Autodesk Inventor part; units mm, degrees
ref_plane "YZ Plane" through (0, 0, 0) normal (1, 0, 0) x (0, 1, 0)
ref_plane "XZ Plane" through (0, 0, 0) normal (0, 1, 0) x (-1, 0, 0)
ref_plane "XY Plane" through (0, 0, 0) normal (0, 0, 1) x (1, 0, 0)
sketch "Sketch1" plane through (0, 0, 0) normal (1, 0, 0) x (0, 1, 0)
  line L0 (0, 0) -> (321.6656, 0)
  line L1 (321.6656, 0) -> (321.6656, 321.6656)
  line L2 (321.6656, 321.6656) -> (0, 321.6656)
  line L3 (0, 321.6656) -> (0, 0)
  dimension "d0" = 321.6656
  dimension "d1" = 321.6656
extrude "Extrusion1" add sketch "Sketch1" along normal blind 4.7752
sketch "Sketch3" plane through (0, 0, 0) normal (-1, 0, 0) x (0, 0, 1)
  line L0 (0, 321.6656) -> (321.6656, 321.6656)
  line L1 (321.6656, 321.6656) -> (321.6656, 0)
  line L2 (0, 321.6656) -> (321.6656, 321.6656)
  line L3 (321.6656, 321.6656) -> (283.5656, 321.6656)
  line L4 (283.5656, 321.6656) -> (283.5656, 283.5656)
  line L5 (283.5656, 283.5656) -> (321.6656, 283.5656)
  line L6 (321.6656, 283.5656) -> (321.6656, 321.6656)
  line L7 (321.6656, 321.6656) -> (321.6656, 0)
  line L8 (321.6656, 0) -> (283.5656, 0)
  line L9 (283.5656, 0) -> (283.5656, 38.1)
  line L10 (283.5656, 38.1) -> (321.6656, 38.1)
  line L11 (321.6656, 38.1) -> (321.6656, 0)
  line L12 (321.6656, 0) -> (0, 0)
  line L13 (0, 0) -> (38.1, 0)
  line L14 (38.1, 0) -> (38.1, 38.1)
  line L15 (38.1, 38.1) -> (0, 38.1)
  line L16 (0, 38.1) -> (0, 0)
  line L17 (0, 321.6656) -> (38.1, 321.6656)
  line L18 (38.1, 321.6656) -> (38.1, 283.5656)
  line L19 (38.1, 283.5656) -> (0, 283.5656)
  line L20 (0, 283.5656) -> (0, 321.6656)
  line L21 (283.5656, 321.6656) -> (38.1, 321.6656)
  line L22 (38.1, 321.6656) -> (38.1, 283.5656)
  line L23 (38.1, 283.5656) -> (283.5656, 283.5656)
  line L24 (283.5656, 283.5656) -> (283.5656, 321.6656)
  line L25 (321.6656, 283.5656) -> (283.5656, 283.5656)
  line L26 (283.5656, 283.5656) -> (283.5656, 38.1)
  line L27 (283.5656, 38.1) -> (321.6656, 38.1)
  line L28 (321.6656, 38.1) -> (321.6656, 283.5656)
  line L29 (38.1, 38.1) -> (0, 38.1)
  line L30 (0, 38.1) -> (0, 283.5656)
  line L31 (0, 283.5656) -> (38.1, 283.5656)
  line L32 (38.1, 283.5656) -> (38.1, 38.1)
  line L33 (38.1, 38.1) -> (283.5656, 38.1)
  line L34 (283.5656, 38.1) -> (283.5656, 0)
  line L35 (283.5656, 0) -> (38.1, 0)
  line L36 (38.1, 0) -> (38.1, 38.1)
  line L37 (321.6656, 283.5656) -> (283.5656, 245.4656)
  line L38 (321.6656, 283.5656) -> (375.5471, 283.5656) construction
  line L39 (283.5656, 245.4656) -> (283.5656, 321.6656)
  line L40 (283.5656, 321.6656) -> (245.4656, 283.5656)
  line L41 (283.5656, 321.6656) -> (337.4471, 321.6656) construction
  line L42 (38.1, 321.6656) -> (76.2, 283.5656)
  line L43 (38.1, 321.6656) -> (91.9815, 321.6656) construction
  line L44 (0, 283.5656) -> (38.1, 245.4656)
  line L45 (0, 283.5656) -> (53.8815, 283.5656) construction
  line L46 (0, 38.1) -> (38.1, 76.2)
  line L47 (0, 38.1) -> (53.8815, 38.1) construction
  line L48 (38.1, 0) -> (76.2, 38.1)
  line L49 (38.1, 0) -> (91.9815, 0) construction
  line L50 (321.6656, 38.1) -> (283.5656, 76.2)
  line L51 (321.6656, 38.1) -> (375.5471, 38.1) construction
  line L52 (283.5656, 0) -> (245.4656, 38.1)
  line L53 (283.5656, 0) -> (337.4471, 0) construction
  dimension "d14" = 38.1
  dimension "d15" = 38.1
  dimension "d16" = 38.1
  dimension "d17" = 38.1
  dimension "d18" = 38.1
  dimension "d19" = 38.1
  dimension "d20" = 38.1
  dimension "d21" = 135
  dimension "d22" = 135
  dimension "d25" = 45
  dimension "d26" = 45
  dimension "d27" = 45
  dimension "d28" = 45
  dimension "d29" = 135
  dimension "d30" = 135
extrude "Extrusion4" cut sketch "Sketch3" against normal blind 4.7752 contours L0 L40 L23 L42 | L44 L32 L46 L30 | L1 L50 L26 L37 | L48 L33 L52 L12
sketch "Sketch4" plane through (0, 0, 0) normal (-1, 0, 0) x (0, 0, 1)
  line L0 (321.6656, 0) -> (283.5656, 0)
  line L1 (321.6656, 38.1) -> (321.6656, 0)
  line L2 (321.6656, 321.6656) -> (321.6656, 283.5656)
  line L3 (283.5656, 321.6656) -> (321.6656, 321.6656)
  line L4 (0, 321.6656) -> (38.1, 321.6656)
  line L5 (0, 283.5656) -> (0, 321.6656)
  line L6 (0, 0) -> (0, 38.1)
  line L7 (38.1, 0) -> (0, 0)
  line L8 (245.4656, 283.5656) -> (283.5656, 321.6656)
  line L9 (283.5656, 321.6656) -> (321.6656, 283.5656)
  line L10 (0, 283.5656) -> (0, 321.6656)
  line L11 (38.1, 321.6656) -> (0, 283.5656)
  line L12 (0, 38.1) -> (38.1, 0)
  line L13 (283.5656, 0) -> (321.6656, 38.1)
extrude "Extrusion5" cut sketch "Sketch4" against normal blind 4.7752
fillet "Fillet1" radius 6.35 16 edges at (2.3876, 283.5656, 0) (2.3876, 321.6656, 38.1) (2.3876, 38.1, 0) (2.3876, 76.2, 38.1) (2.3876, 0, 38.1) (2.3876, 283.5656, 76.2) (2.3876, 283.5656, 245.4656) (2.3876, 321.6656, 283.5656) (2.3876, 283.5656, 321.6656) (2.3876, 76.2, 283.5656) (2.3876, 245.4656, 283.5656) (2.3876, 0, 283.5656) (2.3876, 38.1, 321.6656) (2.3876, 38.1, 76.2) (2.3876, 38.1, 245.4656) (2.3876, 245.4656, 38.1)
sketch "Sketch6" plane through (0, 0, 0) normal (-1, 0, 0) x (0, 0, 1)
  circle A0 centre (-6.7619, -6.7309) radius 6.35
  circle A1 centre (71.9016, 17.9648) radius 6.35
  circle A2 centre (-24.7224, -24.6915) radius 6.35
  circle A3 centre (18.3502, 71.9326) radius 6.35
  circle A4 centre (39.0622, 11.5317) radius 2.159
  circle A5 centre (45.6554, 18.406) radius 2.159
  circle A6 centre (18.4365, 45.0628) radius 2.159
  circle A7 centre (32.185, 31.8764) radius 2.159
  circle A8 centre (11.8433, 38.1885) radius 2.159
  arc A9 (79.2947, 3.1748) -> (87.7766, 8.3381) centre (85.2874, 2.8788) ccw
  line L0 (87.7766, 28.6693) -> (87.7766, 8.3381)
  arc A10 (87.7766, 28.6693) -> (79.2947, 33.8326) centre (85.2874, 34.1286) ccw
  line L1 (40.1516, 33.8326) -> (79.2947, 33.8326)
  arc A11 (33.8016, 40.1826) -> (40.1516, 33.8326) centre (40.1516, 40.1826) ccw
  line L2 (33.8016, 79.3257) -> (33.8016, 40.1826)
  arc A12 (33.8016, 79.3257) -> (28.6383, 87.8076) centre (34.0976, 85.3184) ccw
  line L3 (28.6383, 87.8076) -> (8.3071, 87.8076)
  arc A13 (8.3071, 87.8076) -> (3.1438, 79.3257) centre (2.8478, 85.3184) ccw
  line L4 (3.1438, 27.4834) -> (3.1438, 79.3257)
  arc A14 (1.284, 22.9933) -> (3.1438, 27.4834) centre (-3.2062, 27.4834) ccw
  line L5 (-40.7893, -19.08) -> (1.284, 22.9933)
  arc A15 (-28.7596, -43.1049) -> (-19.111, -40.7583) centre (-23.1391, -45.2051) ccw
  line L6 (22.9623, 1.3149) -> (-19.111, -40.7583)
  arc A16 (27.4524, 3.1748) -> (22.9623, 1.3149) centre (27.4524, -3.1752) ccw
  line L7 (79.2947, 3.1748) -> (27.4524, 3.1748)
  circle A17 centre (85.2874, 34.1286) radius 2.95
  circle A18 centre (2.8478, 85.3184) radius 2.95
  circle A19 centre (-23.1391, -45.2051) radius 2.95
  circle A20 centre (85.2874, 2.8788) radius 2.95
  circle A21 centre (34.0976, 85.3184) radius 2.95
  point P0 (0, 0)
  point P1 (36.9766, 87.8076)
  dimension "d65" = 4.318
extrude "Extrusion7" cut sketch "Sketch6" against normal blind 25.4 contours A4 | A5 | A6 | A7 | A8
sketch "Sketch7" plane through (4.7752, 0, 0) normal (1, 0, 0) x (0, 0, -1)
  circle A0 centre (-31.8764, 289.4806) radius 2.159
  circle A1 centre (-11.5317, 282.6034) radius 2.159
  circle A2 centre (-38.1885, 309.8223) radius 2.159
  circle A3 centre (-18.406, 276.0102) radius 2.159
  circle A4 centre (-45.0628, 303.2291) radius 2.159
  circle A5 centre (-81.9118, 239.7538) radius 19.05
  line L0 (-38.1, 78.8303) -> (-38.1, 242.8353)
  arc A6 (-36.2401, 247.3255) -> (-38.1, 242.8353) centre (-31.75, 242.8353) ccw
  line L1 (-36.2401, 247.3255) -> (-4.4901, 279.0755)
  arc A7 (-4.4901, 279.0755) -> (-4.4901, 288.0557) centre (-8.9803, 283.5656) ccw
  line L2 (-4.4901, 288.0557) -> (-33.6099, 317.1755)
  arc A8 (-33.6099, 317.1755) -> (-42.5901, 317.1755) centre (-38.1, 312.6853) ccw
  line L3 (-42.5901, 317.1755) -> (-74.3401, 285.4255)
  arc A9 (-78.8303, 283.5656) -> (-74.3401, 285.4255) centre (-78.8303, 289.9156) ccw
  line L4 (-78.8303, 283.5656) -> (-242.8353, 283.5656)
  point P0 (0, 0)
  point P1 (-61.0348, 364.3954)
extrude "Extrusion8" cut sketch "Sketch7" against normal blind 25.4 contours A0 | A1 | A2 | A3 | A4
sketch "Sketch8" plane through (4.7752, 0, 0) normal (1, 0, 0) x (0, 0, -1)
  circle A0 centre (-289.7892, 32.185) radius 2.159
  circle A1 centre (-310.1339, 39.0622) radius 2.159
  circle A2 centre (-276.6028, 18.4365) radius 2.159
  circle A3 centre (-303.2596, 45.6554) radius 2.159
  circle A4 centre (-283.4771, 11.8433) radius 2.159
  circle A5 centre (-289.4806, 289.7892) radius 2.159
  circle A6 centre (-282.6034, 310.1339) radius 2.159
  circle A7 centre (-309.8223, 283.4771) radius 2.159
  circle A8 centre (-276.0102, 303.2596) radius 2.159
  circle A9 centre (-303.2291, 276.6028) radius 2.159
  circle A10 centre (-239.7538, 81.9118) radius 19.05
  circle A11 centre (-239.7538, 239.7538) radius 19.05
  line L0 (-78.8303, 283.5656) -> (-242.8353, 283.5656)
  arc A12 (-247.3255, 285.4255) -> (-242.8353, 283.5656) centre (-242.8353, 289.9156) ccw
  line L1 (-247.3255, 285.4255) -> (-279.0755, 317.1755)
  arc A13 (-279.0755, 317.1755) -> (-288.0557, 317.1755) centre (-283.5656, 312.6853) ccw
  line L2 (-288.0557, 317.1755) -> (-317.1755, 288.0557)
  arc A14 (-317.1755, 288.0557) -> (-317.1755, 279.0755) centre (-312.6853, 283.5656) ccw
  line L3 (-317.1755, 279.0755) -> (-285.4255, 247.3255)
  arc A15 (-283.5656, 242.8353) -> (-285.4255, 247.3255) centre (-289.9156, 242.8353) ccw
  line L4 (-283.5656, 242.8353) -> (-283.5656, 78.8303)
  arc A16 (-285.4255, 74.3401) -> (-283.5656, 78.8303) centre (-289.9156, 78.8303) ccw
  line L5 (-285.4255, 74.3401) -> (-317.1755, 42.5901)
  arc A17 (-317.1755, 42.5901) -> (-317.1755, 33.6099) centre (-312.6853, 38.1) ccw
  line L6 (-317.1755, 33.6099) -> (-288.0557, 4.4901)
  arc A18 (-288.0557, 4.4901) -> (-279.0755, 4.4901) centre (-283.5656, 8.9803) ccw
  line L7 (-279.0755, 4.4901) -> (-247.3255, 36.2401)
  arc A19 (-242.8353, 38.1) -> (-247.3255, 36.2401) centre (-242.8353, 31.75) ccw
  line L8 (-242.8353, 38.1) -> (-78.8303, 38.1)
  point P0 (0, 0)
  point P1 (-321.6656, 321.6656)
extrude "Extrusion9" cut sketch "Sketch8" against normal blind 25.4 contours A0 | A1 | A2 | A3 | A4 | A5 | A6 | A7 | A8 | A9
sketch "Sketch9" plane through (4.7752, 0, 0) normal (1, 0, 0) x (0, 0, -1)
  circle A0 centre (-160.8328, 160.8328) radius 19.05
  circle A1 centre (-160.8328, 160.8328) radius 88.9
  circle A2 centre (-160.8328, 249.7328) radius 2.032
  circle A3 centre (-223.6946, 223.6946) radius 2.032
  circle A4 centre (-249.7328, 160.8328) radius 2.032
  circle A5 centre (-223.6946, 97.971) radius 2.032
  circle A6 centre (-160.8328, 71.9328) radius 2.032
  circle A7 centre (-97.971, 97.971) radius 2.032
  circle A8 centre (-71.9328, 160.8328) radius 2.032
  circle A9 centre (-97.971, 223.6946) radius 2.032
  point P0 (0, 0)
  dimension "d54" = 177.8
  dimension "d53" = 38.1
  dimension "d55" = 4.064
  dimension "d61" = 360
extrude "Extrusion10" cut sketch "Sketch9" against normal blind 25.4 contours A1 A8 | A1 A8 | A9 A1 | A1 A9 | A7 A1 | A1 A7 | A2 A1 | A1 A2 | A6 A1 | A1 A6 | A3 A1 | A1 A3 | A5 A1 | A1 A5 | A4 A1 | A1 A4
sketch "Sketch12" plane through (4.7752, 0, 0) normal (1, 0, 0) x (0, 0, -1)
  line L0 (-317.1755, 33.6099) -> (-288.0557, 4.4901)
  line L1 (-33.6099, 4.4901) -> (-4.4901, 33.6099)
  line L2 (-4.4901, 288.0557) -> (-33.6099, 317.1755)
  line L3 (-288.0557, 317.1755) -> (-317.1755, 288.0557)
  line L4 (-302.6156, 302.6156) -> (-19.05, 19.05)
  line L5 (-302.6156, 19.05) -> (-19.05, 302.6156)
  circle A0 centre (-160.8328, 160.8328) radius 12.7
  point P0 (0, 0)
  dimension "d67" = 25.4
extrude "Extrusion11" cut sketch "Sketch12" against normal blind 25.4
sketch "Sketch13" plane through (0, 0, 0) normal (-1, 0, 0) x (0, 0, 1)
  circle A0 centre (160.8328, 160.8328) radius 12.7
  circle A1 centre (160.8328, 116.3828) radius 6.35
  circle A2 centre (160.8328, 160.8328) radius 44.45
  circle A3 centre (199.3276, 138.6078) radius 6.35
  circle A4 centre (199.3276, 183.0578) radius 6.35
  circle A5 centre (160.8328, 205.2828) radius 6.35
  circle A6 centre (122.338, 183.0578) radius 6.35
  circle A7 centre (122.338, 138.6078) radius 6.35
  point P0 (0, 0)
  dimension "d70" = 12.7
  dimension "d71" = 44.45
  dimension "d74" = 360
extrude "Extrusion12" cut sketch "Sketch13" against normal blind 25.4 contours A1 A2 | A2 A1 | A3 A2 | A2 A3 | A7 A2 | A2 A7 | A6 A2 | A2 A6 | A4 A2 | A2 A4 | A5 A2 | A2 A5
properties part number "Frame"
Input: part model. Units: mm. Frame: model coordinates. A direction names the side the tool comes from. Give positions to 0.01 mm unless a question says otherwise; leave off trailing zeros. Order: outer loops, then holes, each group sorted by start corner. A loop starts at its lowest first (then second) coordinate and runs counter-clockwise, first axis right, second up.
1. Draft query along Y for faces 5 (the face through (2.421, 148.435, 163.586)), 6 (the face through (2.354, 18.846, 302.412)), 7 (the face through (2.354, 302.819, 19.254)), 8 (the face through (2.354, 210.637, 164.247)). Return one class per face: released by +Y, released by -Y, zero draft, split by the parting line, or undercut.
Computed:
face 5: undercut
face 6: released by -Y
face 7: released by +Y
face 8: undercut
2. Cut plane B-B (x = 1.35). State how many separate pieces and enclosed holes the cut face has, and give its area (3 significant figures).
Computed:
separate pieces: 1
enclosed holes: 35
area: 67,200 mm2
3. Cut plane A-A (z = 124). Return loops of the section in (x, y), and give its area (3 significant figures).
Computed:
outline: (0, 38.1) - (4.78, 38.1) - (4.78, 132.48) - (0, 132.48) - close; (0, 144.74) - (4.78, 144.74) - (4.78, 176.93) - (0, 176.93) - close; (0, 189.19) - (4.78, 189.19) - (4.78, 283.57) - (0, 283.57) - close
area: 1,060 mm2
4. Cut plane C-C (z = 51.5). Return loops of the section in (x, y), and give its area (3 significant figures).
Computed:
outline: (0, 13.4) - (4.78, 13.4) - (4.78, 308.27) - (0, 308.27) - close
area: 1,410 mm2
5. Cut plane D-D (y = 58.5). Return loops of the section in (x, z), and give its area (3 significant figures).
Computed:
outline: (0, 20.4) - (4.78, 20.4) - (4.78, 301.27) - (0, 301.27) - close
area: 1,340 mm2
6. Set-up query: faces 1 (the face through (2.354, 263.423, 20.143)), 2 (the face through (2.354, 20.143, 263.423)), 3 (the face through (2.354, 301.523, 58.243)), 4 (the face through (2.354, 58.243, 301.523)). Return all of +Z, -Z, +X, -X, +Y, -Y with unobstructed straight access to the full face (end or side cutting, diameter ignored); none if empty.
Computed:
face 1: -Z, +X, -X
face 2: +X, -X, -Y
face 3: +X, -X, +Y
face 4: +Z, +X, -X
7. Pin query (flat end, axial travel): pin 1 Ø1 at (x, z) = (4.5, 207) entering from +Y; pin 2 Ø1 at (x, y) = (3.5, 151.5) entering from -Z; pin 3 Ø2 at (x, y) = (1.5, 258) entering from +Z. Return the tip coordinate at first contact, or that it passes through.
Computed:
pin 1: stops at y = 283.57
pin 2: stops at z = 38.1
pin 3: stops at z = 297.1
8. Line query: probe 1 along Y at (x, z) = (2.35, 223.5); probe 2 along Z at (x, y) = (4.5, 98.5); probe 3 along Z at (x, y) = (4.6, 44). Output: solid intervals per line, ascending.
Computed:
probe 1: y = 38.1 to 95.95, 99.99 to 221.67, 225.72 to 283.57
probe 2: z = 38.1 to 96.01, 99.93 to 221.73, 225.66 to 283.57
probe 3: z = 5.9 to 16.56, 20.32 to 301.87, 304.65 to 315.77
